CAD build for the part. Positions are in the model's coordinates, mm. A direction names the side the tool comes from. Give positions to 0.01 mm unless a question says otherwise; leave off trailing zeros. Order: outer loops, then holes, each group sorted by start corner. A loop starts at its lowest first (then second) coordinate and runs counter-clockwise, first axis right, second up. Notation, with made-up numbers: (60.25, 50.5) -> (98.25, 50.5) arc R19 cw to (98.25, 74.5) -> close; hole circle Ø9 at (12.5, 65.25). An arc over 180 degrees is marked (long way). Use one line per item in the form item = value. Start each with the question number.
1) Mould opens along X. For faces 3 (the face through (10, 3, -62)), 4 (the face through (100.807, 3.131, 67.994)), 5 (the face through (102.938, 3.219, 57.675)), 6 (the face through (-10, 3, -60)) say: pulls with the +X half, pulls with the -X half, needs draft (parallel to the pull), parting line crosses it, or undercut.
2) Cut at B-B, the plane z = 25.5. Give the cut face in (x, y), and give its area (3 significant figures).
3) Drop flat-ended pins along their axis: P1, Ø2, axis at y = 5, z = -50.5, coming from the -X side; P2, Ø3, axis at x = -10, y = 5.5, coming from the +Z side; P3, Ø1.5, axis at y = 4.5, z = -16, coming from the +X side; P4, Ø6, axis at x = -100.46, z = 58, coming from the +Y side. Give the stop position or say it passes through.
4) Probe line 1 (X direction, y = 1.75, z = 58); line 2 (X direction, y = 2, z = -67); line 3 (X direction, y = 2.25, z = 54). List the from-to ranges inside material, lowest first.
5) Cut at A-A, the plane y = 2.25. Give the cut face in (x, z), and give its area (3 significant figures).
6) Cut at C-C, the plane z = -11. Give the cut face in (x, y), and give its area (3 significant figures).
7) Cut at D-D, the plane x = -91. Give the cut face in (y, z).
8) Tool access for faces 1 (the face through (48.4, 3.13, 39.49)), 2 (the face through (-58.4, 3.13, 22.17)): list every direction of +Z, -Z, +X, -X, +Y, -Y with a clear straight run to the whole face (end or side of a thin tool).
from build123d import *

# Parameters (mm, degrees)
SKETCH1_R           = 125
BOSS_EXTRUDE1_DEPTH = 6.35
SKETCH2_R           = 2.5
CUT_EXTRUDE1_DEPTH  = 177.890707783
CUT_EXTRUDE2_START  = -10
CUT_EXTRUDE2_DEPTH  = 10


with BuildPart() as part:
    # Sketch1 → Boss-Extrude1 (new body)
    with BuildSketch(Plane(origin=(0, 0, 0), x_dir=(1, 0, 0), z_dir=(0, 1, 0))):
        with Locations(Location((0, 0, 0), (0, 0, 270))):
            Circle(SKETCH1_R)
    extrude(amount=BOSS_EXTRUDE1_DEPTH)

    # Sketch2 → Cut-Extrude1 (cut, through all)
    with BuildSketch(Plane(origin=(0, 6.35, 0), x_dir=(1, 0, 0), z_dir=(0, 1, 0))):
        with Locations(Location((0, 116, 0), (0, 0, 270))):
            Circle(SKETCH2_R)
        with Locations(Location((100.458946839, -58, 0), (0, 0, 270))):
            Circle(SKETCH2_R)
        with Locations(Location((-100.458946839, -58, 0), (0, 0, 270))):
            Circle(SKETCH2_R)
    extrude(amount=-CUT_EXTRUDE1_DEPTH, mode=Mode.SUBTRACT)

    # Sketch6 → Cut-Extrude2 (cut)
    with BuildSketch(Plane(origin=(0, 6.35, 0), x_dir=(1, 0, 0), z_dir=(0, 1, 0)).offset(CUT_EXTRUDE2_START)):
        with BuildLine():
            ThreePointArc((-10, 116), (-8.52176463, 121.232545039), (-4.524094482, 124.918103448))
            ThreePointArc((-4.524094482, 124.918103448), (-108.253175473, 62.5), (-110.44429822, -58.541070973))
            ThreePointArc((-110.44429822, -58.541070973), (-109.251346085, -53.236207865), (-105.458946839, -49.339745962))
            Line((-105.458946839, -49.339745962), (-10, 5.773502692))
            Line((-10, 5.773502692), (-10, 116))
        make_face()
        with BuildLine():
            ThreePointArc((4.524094482, 124.918103448), (8.52176463, 121.232545039), (10, 116))
            Line((10, 116), (10, 5.773502692))
            Line((10, 5.773502692), (105.458946839, -49.339745962))
            ThreePointArc((105.458946839, -49.339745962), (109.251346085, -53.236207865), (110.44429822, -58.541070973))
            ThreePointArc((110.44429822, -58.541070973), (121.306506993, -30.161753285), (125, 0))
            ThreePointArc((125, 0), (89.973640057, 86.774098064), (4.524094482, 124.918103448))
        make_face()
        with BuildLine():
            Line((95.458946839, -66.660254038), (0, -11.547005384))
            Line((0, -11.547005384), (-95.458946839, -66.660254038))
            ThreePointArc((-95.458946839, -66.660254038), (-100.729581454, -67.996337174), (-105.920203738, -66.377032475))
            ThreePointArc((-105.920203738, -66.377032475), (0, -125), (105.920203738, -66.377032475))
            ThreePointArc((105.920203738, -66.377032475), (100.729581454, -67.996337174), (95.458946839, -66.660254038))
        make_face()
    extrude(amount=CUT_EXTRUDE2_DEPTH, mode=Mode.SUBTRACT)


solid = part.part
Result:
q1.face_3 = pulls with the +X half
q1.face_4 = undercut
q1.face_5 = undercut
q1.face_6 = pulls with the -X half
q2.outline = (-64.17, 0) -> (-24.17, 0) -> (-24.17, 6.35) -> (-64.17, 6.35) -> close; (24.17, 0) -> (64.17, 0) -> (64.17, 6.35) -> (24.17, 6.35) -> close
q2.area = 508 mm²
q3.P1 = -10
q3.P2 = 18.19
q3.P3 = 10
q3.P4 = 6.35
q4.line_1 = -110.46 to -102.96, -97.96 to -80.46, 80.46 to 97.96, 102.96 to 110.46
q4.line_2 = -10 to 10
q4.line_3 = -109.62 to -73.53, 73.53 to 109.62
q5.outline = (-110.44, 58.54) arc R10 ccw to (-105.46, 49.34) -> (-10, -5.77) -> (-10, -116) arc R10 ccw to (-4.52, -124.92) arc R125 ccw to (4.52, -124.92) arc R10 ccw to (10, -116) -> (10, -5.77) -> (105.46, 49.34) arc R10 ccw to (110.44, 58.54) arc R125 ccw to (105.92, 66.38) arc R10 ccw to (95.46, 66.66) -> (0, 11.55) -> (-95.46, 66.66) arc R10 ccw to (-105.92, 66.38) arc R125 ccw to start; hole circle Ø5 at (-100.46, 58); hole circle Ø5 at (0, -116); hole circle Ø5 at (100.46, 58)
q5.area = 7,180 mm²
q6.outline = (-10, 0) -> (10, 0) -> (10, 6.35) -> (-10, 6.35) -> close
q6.area = 127 mm²
q7.outline = (0, 40.99) -> (6.35, 40.99) -> (6.35, 64.09) -> (0, 64.09) -> close
q8.face_1 = +Z, +Y, -Y
q8.face_2 = -Z, -X, +Y, -Y
